```python
from build123d import *

# Parameters (mm, degrees)
EXTRUDE1_DEPTH = 3.175
EXTRUDE2_DEPTH = 94.295303002


with BuildPart() as part:
    # Sketch1 → Extrude1 (new body)
    with BuildSketch(Plane.XY):
        with BuildLine():
            Line((-18.257091065, 0), (2.640813879, 0))
            ThreePointArc((2.640813879, 0), (4.430938656, 0.552772267), (5.59773661, 2.018612104))
            Line((5.59773661, 2.018612104), (28.983052402, 61.815650828))
            ThreePointArc((28.983052402, 61.815650828), (28.648357405, 64.762163501), (26.026129672, 66.147038724))
            Line((26.026129672, 66.147038724), (-18.257091065, 66.147038724))
            Line((-18.257091065, 66.147038724), (-18.257091065, 0))
        make_face()
    extrude(amount=-EXTRUDE1_DEPTH)

    # Mirror1: part across plane


with BuildPart() as part_1:
    add(part.part)
    add(part.part.mirror(Plane(origin=(-18.257091065, 66.147038724, -3.175), x_dir=(0, 0, 1), z_dir=(-1, 0, 0))))

    # Sketch2 → Extrude2 (cut, through all)
    with BuildSketch(Plane.XY):
        with BuildLine():
            Line((0.725945487, 6.995955873), (1.798751091, 9.739155873))
            ThreePointArc((1.798751091, 9.739155873), (1.691648692, 10.682039928), (0.852535818, 11.1252))
            Line((0.852535818, 11.1252), (-37.366717948, 11.1252))
            ThreePointArc((-37.366717948, 11.1252), (-38.205830822, 10.682039928), (-38.312933221, 9.739155873))
            Line((-38.312933221, 9.739155873), (-37.240127617, 6.995955873))
            ThreePointArc((-37.240127617, 6.995955873), (-36.866752272, 6.526887125), (-36.293912343, 6.35))
            Line((-36.293912343, 6.35), (-0.220269787, 6.35))
            ThreePointArc((-0.220269787, 6.35), (0.352570142, 6.526887125), (0.725945487, 6.995955873))
        make_face()
    extrude(amount=-EXTRUDE2_DEPTH, mode=Mode.SUBTRACT)


solid = part_1.part
```
Verification items for the finished model (mm, model axes). A direction names the side the tool comes from. Round coordinates to 2 decimals unless told otherwise and drop trailing zeros. Write each loop counter-clockwise with the first axis right and the second up, starting at its lowest first coordinate (ties: lowest second). Pieces come first, ordered by that corner, then holes. Notation, with made-up numbers: (-8.75, 72.5) - (15.25, 72.5) arc R14 ccw to (15.25, 80.5) - close; hole circle Ø7 at (-30, 72). An arc over 180 degrees is marked (long way). Answer as a JSON object with one key per item and string values. Group by question number.
Q1. Section check B-B, the plane z = -1.75. Enter the section's corners in (x, y) (3 decimals), plus the area to 3 significant figures.
Q2. Mould release check, pull along X, two halves, no side actions. Record for faces 3 (the flat face through (-19, 66.147, -2)), 4 (the cylindrical face through (28.67, 64.73, -1.57)), 5 (the flat face through (1.255, 8.348, -1.565)): released by +X, released by -X, zero draft, split by the parting line, or undercut.
Q3. Thickness scan on line 1 (Y direction, x = -13, z = -2.6); line 2 (X direction, y = 40.5, z = -2.9); line 3 (X direction, y = 51, z = -2.9). Record the ranges inside material, lowest first.
Q4. Section check C-C, the plane y = 21. Enter the section's corners in (x, z) (3 decimals), plus the area to 3 significant figures.
Q5. Tool access check on faces 1 (the flat face through (-19, 6.35, -2)), 2 (the flat face through (-18, 41, 0)). Record the directions out of +Z, -Z, +X, -X, +Y, -Y that give a thin tool (end or side, any length) a straight path to the whole face; none if there is none.
Q6. Section check D-D, the plane x = 17. Enter the section's corners in (y, z) (3 decimals), plus the area to 3 significant figures.
Q7. Section check A-A, the plane x = -24.5. Enter the section's corners in (y, z) (3 decimals), plus the area to 3 significant figures.
Found:
{
 "1": {"outline": "(-65.497, 61.816) - (-42.112, 2.019) arc R3.175 ccw to (-39.155, 0) - (2.641, 0) arc R3.175 ccw to (5.598, 2.019) - (28.983, 61.816) arc R3.175 ccw to (26.026, 66.147) - (-62.54, 66.147) arc R3.175 ccw to start; hole (-38.313, 9.739) - (-37.24, 6.996) arc R1.016 ccw to (-36.294, 6.35) - (-0.22, 6.35) arc R1.016 ccw to (0.726, 6.996) - (1.799, 9.739) arc R1.016 ccw to (0.853, 11.125) - (-37.367, 11.125) arc R1.016 ccw to start", "area": "4,560 mm^2"},
 "2": {"face 3": "zero draft", "face 4": "released by +X", "face 5": "undercut"},
 "3": {"line 1": "y = 0 to 6.35, 11.13 to 66.15", "line 2": "x = -57.16 to 20.65", "line 3": "x = -61.27 to 24.75"},
 "4": {"outline": "(-49.535, -3.175) - (13.021, -3.175) - (13.021, 0) - (-49.535, 0) - close", "area": "199 mm^2"},
 "5": {"face 1": "+Z, -Z", "face 2": "+Z, +X, -X, +Y, -Y"},
 "6": {"outline": "(31.175, -3.175) - (66.147, -3.175) - (66.147, 0) - (31.175, 0) - close", "area": "111 mm^2"},
 "7": {"outline": "(0, -3.175) - (6.35, -3.175) - (6.35, 0) - (0, 0) - close; (11.125, -3.175) - (66.147, -3.175) - (66.147, 0) - (11.125, 0) - close", "area": "195 mm^2"}
}
